Work out the finished part from the listing and answer in its coordinate system (mm). A direction names the side the tool comes from. Give positions to 0.01 mm unless a question says otherwise; leave off trailing zeros. Loops run counter-clockwise (first coordinate to the right, second up) from the corner with the lowest first, then second, coordinate; pieces in that order, holes last. Notation, with made-up numbers: M 80.5,-15.5 L 124.5,-15.5 A10 cw 124.5,-3.5 Z; hole C -25.75,-8.5 d9. An arc over 180 degrees is marked long. Answer in a Markdown table with one row per item. Add a question column.
from build123d import *

# Parameters (mm, degrees)
CUT_EXTRUDE1_DEPTH      = 33.691742077
CUT_EXTRUDE1_DEPTH_BACK = 33.691742077
SKETCH3_R               = 2
SKETCH3_R_2             = 1


with BuildPart() as part:
    # Sketch2 → Revolve1 (revolve)
    with BuildSketch(Plane.XY, mode=Mode.PRIVATE) as revolve1_sk:
        Polygon((7.5, 13.9), (-7.5, 13.9), (-7.5, 16.9), (-2.692932377, 16.9), (-2.692932377, 19.9), (-4.5, 19.9), (-4.5, 22.5), (4.5, 22.5), (4.5, 19.9), (2.692932377, 19.9), (2.692932377, 16.9), (7.5, 16.9), align=None)
    revolve(revolve1_sk.sketch.rotate(Axis((-32.720414201, 0, 0), (1, 0, 0)), 90), axis=Axis((-32.720414201, 0, 0), (1, 0, 0)))

    # Sketch3 → Cut-Extrude1 (cut, two sides: drawn at the far end of the back side and taken through both)
    with BuildSketch(Plane(origin=(0, 0, 0), x_dir=(0, 0, -1), z_dir=(1, 0, 0)).offset(-CUT_EXTRUDE1_DEPTH_BACK)):
        with Locations((7.292672674, 22.444538631)):
            Circle(SKETCH3_R)
        with Locations((-2.904929565, 18.34100344)):
            Circle(SKETCH3_R_2)
        with Locations((13.871487736, 19.09246493)):
            Circle(SKETCH3_R)
        with Locations((19.09246493, 13.871487736)):
            Circle(SKETCH3_R)
        with Locations((22.444538631, 7.292672674)):
            Circle(SKETCH3_R)
        with Locations((23.599584511, 0)):
            Circle(SKETCH3_R)
        with Locations((22.444538631, -7.292672674)):
            Circle(SKETCH3_R)
        with Locations((19.09246493, -13.871487736)):
            Circle(SKETCH3_R)
        with Locations((13.871487736, -19.09246493)):
            Circle(SKETCH3_R)
        with Locations((7.292672674, -22.444538631)):
            Circle(SKETCH3_R)
        with Locations((0, -23.599584511)):
            Circle(SKETCH3_R)
        with Locations((-7.292672674, -22.444538631)):
            Circle(SKETCH3_R)
        with Locations((-13.871487736, -19.09246493)):
            Circle(SKETCH3_R)
        with Locations((-19.09246493, -13.871487736)):
            Circle(SKETCH3_R)
        with Locations((-22.444538631, -7.292672674)):
            Circle(SKETCH3_R)
        with Locations((-23.599584511, 0)):
            Circle(SKETCH3_R)
        with Locations((-22.444538631, 7.292672674)):
            Circle(SKETCH3_R)
        with Locations((-19.09246493, 13.871487736)):
            Circle(SKETCH3_R)
        with Locations((-13.871487736, 19.09246493)):
            Circle(SKETCH3_R)
        with Locations((-7.292672674, 22.444538631)):
            Circle(SKETCH3_R)
        with Locations((0, 23.599584511)):
            Circle(SKETCH3_R)
        with Locations((2.904929565, 18.34100344)):
            Circle(SKETCH3_R_2)
        with Locations((8.430433949, 16.545658234)):
            Circle(SKETCH3_R_2)
        with Locations((13.13070872, 13.13070872)):
            Circle(SKETCH3_R_2)
        with Locations((16.545658234, 8.430433949)):
            Circle(SKETCH3_R_2)
        with Locations((18.34100344, 2.904929565)):
            Circle(SKETCH3_R_2)
        with Locations((18.34100344, -2.904929565)):
            Circle(SKETCH3_R_2)
        with Locations((16.545658234, -8.430433949)):
            Circle(SKETCH3_R_2)
        with Locations((13.13070872, -13.13070872)):
            Circle(SKETCH3_R_2)
        with Locations((8.430433949, -16.545658234)):
            Circle(SKETCH3_R_2)
        with Locations((2.904929565, -18.34100344)):
            Circle(SKETCH3_R_2)
        with Locations((-2.904929565, -18.34100344)):
            Circle(SKETCH3_R_2)
        with Locations((-8.430433949, -16.545658234)):
            Circle(SKETCH3_R_2)
        with Locations((-13.13070872, -13.13070872)):
            Circle(SKETCH3_R_2)
        with Locations((-16.545658234, -8.430433949)):
            Circle(SKETCH3_R_2)
        with Locations((-18.34100344, -2.904929565)):
            Circle(SKETCH3_R_2)
        with Locations((-18.34100344, 2.904929565)):
            Circle(SKETCH3_R_2)
        with Locations((-16.545658234, 8.430433949)):
            Circle(SKETCH3_R_2)
        with Locations((-13.13070872, 13.13070872)):
            Circle(SKETCH3_R_2)
        with Locations((-8.430433949, 16.545658234)):
            Circle(SKETCH3_R_2)
    extrude(amount=CUT_EXTRUDE1_DEPTH + CUT_EXTRUDE1_DEPTH_BACK, mode=Mode.SUBTRACT)


solid = part.part
(1) Section A-A, the plane y = 0 is taken. Determine the outline of the cut face in (x, z), and give its area (3 significant figures).
(2) Section D-D, the plane x = -1.75 is taken. State how many separate pieces and enclosed holes the cut face has, and give its area (3 significant figures).
(3) Which of the six approach directions +Z, -Z, +X, -X, +Y, -Y give full straight-line access (tool end or side, diameter ignored) to faces 1 (the face through (5.13, -5.08, 16.12)), 2 (the face through (-0.06, -6.65, -20.55)), 3 (the face through (-3.6, 12.1, -15.8))?
(4) Consider line 1 along Y through (x, z) = (-2.75, -7.5); line 2 along Z through (x, y) = (-0.25, -2); line 3 along Z through (x, y) = (-2.75, 4.5). Determine where each line is inside the solid, lowest interval first. Write a range as from..to.
(5) Each of these flat-tipped pins is pushed along its axis until it touches: P1, Ø4, axis at x = 2, y = -13, coming from the -Z side; P2, Ø3, axis at y = 16.55, z = -8.43, coming from the -X side; P3, Ø2.5, axis at y = 18.34, z = -2.9, coming from the +X side. Where does it stop, or does it pass through?
(6) Section C-C, the plane x = -6.25 is taken. Determine the outline of the cut face in (y, z), and give its area (3 significant figures).
(7) The mould has two halves that part along Y. Classify faces 4 (the face through (-0.038, 7.454, 16.762)), 5 (the face through (0.06, 15.89, -15.93)), 6 (the face through (7.5, 14, 2)): pulls with the +Y half, pulls with the -Y half, needs draft (parallel to the pull), parting line crosses it, or undercut.
Numbers:
| question | item | result |
|---|---|---|
| 1 | outline | M -7.5,-16.9 L -2.69,-16.9 L -2.69,-19.9 L -4.5,-19.9 L -4.5,-21.6 L 4.5,-21.6 L 4.5,-19.9 L 2.69,-19.9 L 2.69,-16.9 L 7.5,-16.9 L 7.5,-13.9 L -7.5,-13.9 Z; M -7.5,13.9 L 7.5,13.9 L 7.5,16.9 L 2.69,16.9 L 2.69,19.9 L 4.5,19.9 L 4.5,21.6 L -4.5,21.6 L -4.5,19.9 L -2.69,19.9 L -2.69,16.9 L -7.5,16.9 Z |
| 1 | area | 153 mm² |
| 2 | separate pieces | 1 |
| 2 | enclosed holes | 21 |
| 2 | area | 880 mm² |
| 3 | face 1 | +X |
| 3 | face 2 | -Z, +X, -X |
| 3 | face 3 | -X |
| 4 | line 1 | y = -20.46..-18.43, -15.14..-11.7, 11.7..15.14, 18.43..20.46 |
| 4 | line 2 | z = -22.41..-18.77, -17.92..-13.76, 13.76..17.92, 18.77..22.41 |
| 4 | line 3 | z = -22.05..-19.38, -16.29..-13.15, 13.15..16.29, 19.38..22.05 |
| 5 | P1 | stops at z = -19.63 |
| 5 | P2 | stops at x = -4.5 |
| 5 | P3 | stops at x = 2.69 |
| 6 | outline | C 0,0 d33.8; hole C 0,0 d27.8 |
| 6 | area | 290 mm² |
| 7 | face 4 | undercut |
| 7 | face 5 | pulls with the +Y half |
| 7 | face 6 | needs draft |
